```python
from build123d import *

# Parameters (mm, degrees)
PAD_DEPTH     = 5
SKETCH001_R   = 1.7
HOLE_DEPTH    = 72.8243
SKETCH002_W   = 30
SKETCH002_H   = 5
PAD001_DEPTH  = 10.1
SKETCH003_W   = 10
SKETCH003_H   = 30
PAD002_DEPTH  = 20
SKETCH005_R   = 3.55
HOLE001_DEPTH = 10.001
POCKET_DEPTH  = 30.001
FILLET_R      = 10


with BuildPart() as part:
    # Sketch → Pad (new body)
    with BuildSketch(Plane.XY):
        with BuildLine():
            Line((-15, 0), (0, 0))
            Line((0, 0), (0, 15))
            Line((0, 15), (-10, 15))
            ThreePointArc((-10, 15), (-13.535534, 13.535534), (-15, 10))
            Line((-15, 10), (-15, 0))
        make_face()
    pad = extrude(amount=PAD_DEPTH)

    # Mirrored: Pad across XZ
    add(pad.mirror(Plane.XZ))

    # Sketch001 (on Face5 of Mirrored) → Hole (cut, through all)
    with BuildSketch(Plane.XY.offset(5)):
        with Locations((-7.5, 7.5)):
            Circle(SKETCH001_R)
    hole = extrude(amount=-HOLE_DEPTH, mode=Mode.SUBTRACT)

    # Mirrored001: Hole across XZ
    add(hole.mirror(Plane.XZ), mode=Mode.SUBTRACT)

    # Sketch002 (on Face2 of Mirrored001) → Pad001 (join)
    with BuildSketch(Plane.YZ):
        with Locations((0, 2.5)):
            Rectangle(SKETCH002_W, SKETCH002_H)
    extrude(amount=PAD001_DEPTH)

    # Sketch003 (on Face7 of Pad001) → Pad002 (join)
    with BuildSketch(Plane.XY.offset(5)):
        with Locations((5.1, 0)):
            Rectangle(SKETCH003_W, SKETCH003_H)
    extrude(amount=PAD002_DEPTH)

    # Sketch005 (on Face15 of Pad002) → Hole001 (cut, through all)
    with BuildSketch(Plane(origin=(0.1, 0, 0), x_dir=(0, -1, 0), z_dir=(-1, 0, 0))):
        with Locations((0, 15)):
            Circle(SKETCH005_R)
    extrude(amount=-HOLE001_DEPTH, mode=Mode.SUBTRACT)

    # Sketch006 (on Face14 of Hole001) → Pocket (cut, through all)
    with BuildSketch(Plane.XZ.offset(15)):
        with BuildLine():
            ThreePointArc((10.1, 3), (7.97868, 2.12132), (7.1, 0))
            Line((10.1, 0), (7.1, 0))
            Line((10.1, 3), (10.1, 0))
        make_face()
    extrude(amount=-POCKET_DEPTH, mode=Mode.SUBTRACT)

    # Fillet
    fillet_edges = [part.edges().sort_by_distance(p)[0] for p in [
        (5.1, -15, 25),
        (5.1, 15, 25),
    ]]
    fillet(fillet_edges, radius=FILLET_R)


solid = part.part
```
Build history of the part. All positions in model axes, mm. A direction names the side the tool comes from. Give positions to 0.01 mm unless a question says otherwise; leave off trailing zeros. Loops run counter-clockwise (first coordinate to the right, second up) from the corner with the lowest first, then second, coordinate; pieces in that order, holes last. Notation, with made-up numbers: (53.5, 89.25) -> (112.5, 89.25) arc R33 cw to (112.5, 123.25) -> close; hole circle Ø7 at (11, 84.25). An arc over 180 degrees is marked (long way). One line per question, with ' | ' between items. Start each with the question number.
1) Cut at C-C (z = 16). Give the cut face in (x, y).
2) Pin check, flat tips, straight feed: pin 1 (4.5 mm diameter, centred on x = -6, y = -7, fed in from +Z); pin 2 (6 mm diameter, centred on y = -4.5, z = 15.5, fed in from -X); pin 3 (2 mm diameter, centred on y = -11, z = 2.5, fed in from +X). Stop position of each tip, or through.
3) Two-plate mould, pull along X, no slides. Class faces 1 (the cylindrical face through (5.17, 11.99, 22.15)), 2 (the cylindrical face through (-7.87, -5.84, 2.54)), 3 (the cylindrical face through (8, -0.21, 2.14)), 4 (the cylindrical face through (-7.87, 5.84, 2.54)): released by +X, released by -X, zero draft, split by the parting line, or undercut.
4) Cut at A-A (y = 0). Give the cut face in (x, z).
5) Cut at B-B (x = -7.5). Give the cut face in (y, z).
6) 3-axis set-ups, long thin cutter, end or side, ignore diameter. For faces 5 (the flat face through (0.1, 3.1, 12.6)), 6 (the cylindrical face through (-13, 14, 2)): which of +Z, -Z, +X, -X, +Y, -Y reach the whole face in a straight line?
7) Probe L1, parallel to Y at x = -7.5, z = 2.4; L2, parallel to Z at x = 4.5, y = 0; L3, parallel to Z at x = -12, y = 13. List the from-to ranges inside material, lowest first.
8) Cut at D-D (x = 0.75). Give the cut face in (y, z).
Return value:
1) outline: (0.1, -14.95) -> (10.1, -14.95) -> (10.1, -3.41) -> (0.1, -3.41) -> close; (0.1, 3.41) -> (10.1, 3.41) -> (10.1, 14.95) -> (0.1, 14.95) -> close
2) pin 1: z = 5 | pin 2: x = 0.1 | pin 3: x = 10.1
3) face 1: zero draft | face 2: undercut | face 3: released by +X | face 4: undercut
4) outline: (-15, 0) -> (7.1, 0) arc R3 cw to (10.1, 3) -> (10.1, 11.45) -> (0.1, 11.45) -> (0.1, 5) -> (-15, 5) -> close; (0.1, 18.55) -> (10.1, 18.55) -> (10.1, 25) -> (0.1, 25) -> close
5) outline: (-15, 0) -> (-9.2, 0) -> (-9.2, 5) -> (-15, 5) -> close; (-5.8, 0) -> (5.8, 0) -> (5.8, 5) -> (-5.8, 5) -> close; (9.2, 0) -> (15, 0) -> (15, 5) -> (9.2, 5) -> close
6) face 5: +Z, -X, +Y, -Y | face 6: +Z, -Z, -X, +Y
7) L1: -15 to -9.2, -5.8 to 5.8, 9.2 to 15 | L2: 0 to 11.45, 18.55 to 25 | L3: 0 to 5
8) outline: (-15, 0) -> (15, 0) -> (15, 15) arc R10 ccw to (5, 25) -> (-5, 25) arc R10 ccw to (-15, 15) -> close; hole circle Ø7.1 at (0, 15)
